Read the model definition and answer for the solid it produces. Units are mm, in the model's axes. Face numbers are marked on the shaded views. A direction names the side the tool comes from. Give positions to 0.01 mm unless a question says otherwise; leave off trailing zeros. Loops run counter-clockwise (first coordinate to the right, second up) from the corner with the lowest first, then second, coordinate; pieces in that order, holes last. Notation, with made-up numbers: (8, 57.25) -> (55, 57.25) arc R8 cw to (55, 62.25) -> close; hole circle Ø5 at (9, -30). An arc over 180 degrees is marked (long way). One line per item, written item: value. Start each with the question number.
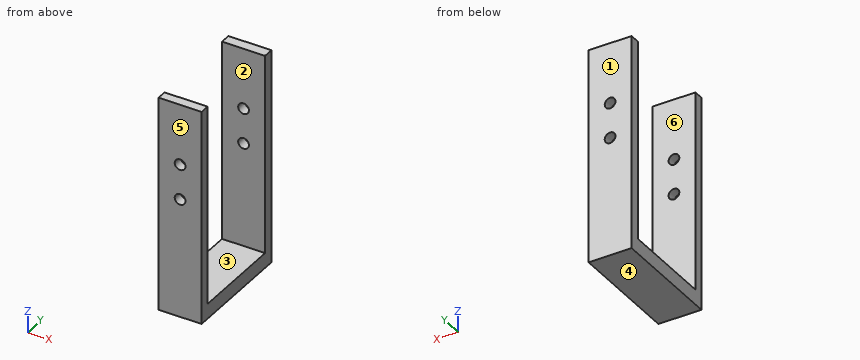
from build123d import *

# Parameters (mm, degrees)
SKETCH1_W           = 20
SKETCH1_H           = 100
BOSS_EXTRUDE1_DEPTH = 53
SKETCH2_W           = 20
SKETCH2_H           = 22.115254232
CUT_EXTRUDE1_DEPTH  = 93
SKETCH4_W           = 20
SKETCH4_H           = 7.428579278
CUT_EXTRUDE3_DEPTH  = 93
SKETCH5_W           = 20
SKETCH5_H           = 14.111734172
CUT_EXTRUDE4_DEPTH  = 93
SKETCH6_R           = 2.5
CUT_EXTRUDE5_DEPTH  = 70
SKETCH8_R           = 2.5
CUT_EXTRUDE7_DEPTH  = 67


with BuildPart() as part:
    # Sketch1 → Boss-Extrude1 (new body)
    with BuildSketch(Plane(origin=(0, 0, 0), x_dir=(1, 0, 0), z_dir=(0, 1, 0))):
        Rectangle(SKETCH1_W, SKETCH1_H)
    extrude(amount=BOSS_EXTRUDE1_DEPTH)

    # Sketch2 → Cut-Extrude1 (cut)
    with BuildSketch(Plane.XY.offset(50)):
        with Locations((0, 15.581680587)):
            Rectangle(SKETCH2_W, SKETCH2_H)
    extrude(amount=-CUT_EXTRUDE1_DEPTH, mode=Mode.SUBTRACT)

    # Sketch4 → Cut-Extrude3 (cut)
    with BuildSketch(Plane.XY.offset(50)):
        with Locations((0, 30.353597342)):
            Rectangle(SKETCH4_W, SKETCH4_H)
    extrude(amount=-CUT_EXTRUDE3_DEPTH, mode=Mode.SUBTRACT)

    # Sketch5 → Cut-Extrude4 (cut)
    with BuildSketch(Plane.XY.offset(50)):
        with Locations((0, 41.123754067)):
            Rectangle(SKETCH5_W, SKETCH5_H)
    extrude(amount=-CUT_EXTRUDE4_DEPTH, mode=Mode.SUBTRACT)

    # Sketch6 → Cut-Extrude5 (cut)
    with BuildSketch(Plane(origin=(0, 53, 0), x_dir=(1, 0, 0), z_dir=(0, 1, 0))):
        with Locations(Location((0, -5.385612406, 0), (0, 0, 270))):
            Circle(SKETCH6_R)
    extrude(amount=-CUT_EXTRUDE5_DEPTH, mode=Mode.SUBTRACT)

    # Sketch8 → Cut-Extrude7 (cut)
    with BuildSketch(Plane(origin=(0, 53, 0), x_dir=(1, 0, 0), z_dir=(0, 1, 0))):
        with Locations(Location((0, -21.748837603, 0), (0, 0, 270))):
            Circle(SKETCH8_R)
    extrude(amount=-CUT_EXTRUDE7_DEPTH, mode=Mode.SUBTRACT)


solid = part.part
Item 1: Section C-C, the plane x = -7.5 is taken. Determine the outline of the cut face in (y, z).
Item 2: Determine the mould class of the marked faces 1, 2, 3 and 4 for opening direction Y: pulls with the +Y half, pulls with the -Y half, needs draft (parallel to the pull), parting line crosses it, or undercut.
Item 3: Section B-B, the plane x = 0 is taken. Determine the outline of the cut face in (y, z), plus the area to 3 significant figures.
Item 4: For the marked faces 5 and 6, determine the directions among +Z, -Z, +X, -X, +Y, -Y from which every point of the face is accessible in a straight line to the end or side of a thin tool.
Item 5: Consider L1, parallel to Y at x = 3.5, z = 37.5; L2, parallel to Z at x = 7.5, y = 6.5. Determine where each line is inside the solid, lowest interval first. Write a range as [from, to].
Item 6: Section D-D, the plane y = 33 is taken. Determine the outline of the cut face in (x, z), plus the area to 3 significant figures.
Item 7: Section A-A, the plane z = -30 is taken. Determine the outline of the cut face in (x, y), plus the area to 3 significant figures.
Item 8: Flat-ended cylindrical pins translate along their axes: pin 1 (4 mm diameter, centred on x = 0, z = 5.39, fed in from -Y); pin 2 (8 mm diameter, centred on x = -7, y = 9, fed in from +Z). Find the tip coordinate at first contact, or state that the pin passes through.
Computed values:
1. outline: (0, -50) -> (53, -50) -> (53, 50) -> (48.18, 50) -> (48.18, -43) -> (4.52, -43) -> (4.52, 50) -> (0, 50) -> close
2. face 1: pulls with the +Y half
2. face 2: undercut
2. face 3: undercut
2. face 4: needs draft
3. outline: (0, -50) -> (53, -50) -> (53, 2.89) -> (48.18, 2.89) -> (48.18, -43) -> (4.52, -43) -> (4.52, 2.89) -> (0, 2.89) -> close; (0, 7.89) -> (4.52, 7.89) -> (4.52, 19.25) -> (0, 19.25) -> close; (0, 24.25) -> (4.52, 24.25) -> (4.52, 50) -> (0, 50) -> close; (48.18, 7.89) -> (53, 7.89) -> (53, 19.25) -> (48.18, 19.25) -> close; (48.18, 24.25) -> (53, 24.25) -> (53, 50) -> (48.18, 50) -> close
3. area: 1,150 mm²
4. face 5: +Z, -Z, +X, -X, -Y
4. face 6: +Z, +X, -X
5. L1: [0, 4.52], [48.18, 53]
5. L2: [-50, -43]
6. outline: (-10, -50) -> (10, -50) -> (10, -43) -> (-10, -43) -> close
6. area: 140 mm²
7. outline: (-10, 0) -> (10, 0) -> (10, 4.52) -> (-10, 4.52) -> close; (-10, 48.18) -> (10, 48.18) -> (10, 53) -> (-10, 53) -> close
7. area: 187 mm²
8. pin 1: through
8. pin 2: z = -43
